from build123d import *

# Parameters (mm, degrees)
SKETCH2_W           = 127
SKETCH2_H           = 60
SKETCH2_W_2         = 105
SKETCH2_H_2         = 41
BOSS_EXTRUDE2_DEPTH = 8
SKETCH3_R           = 2.15
CUT_EXTRUDE1_DEPTH  = 5.159375
SKETCH4_W           = 11
SKETCH4_H           = 9.5
BOSS_EXTRUDE3_DEPTH = 25


with BuildPart() as part:
    # Sketch2 → Boss-Extrude2 (new body)
    with BuildSketch(Plane(origin=(0, 0, 0), x_dir=(1, 0, 0), z_dir=(0, 1, 0))):
        Rectangle(SKETCH2_W, SKETCH2_H)
        Rectangle(SKETCH2_W_2, SKETCH2_H_2, mode=Mode.SUBTRACT)
    extrude(amount=-BOSS_EXTRUDE2_DEPTH)

    # Sketch3 → Cut-Extrude1 (cut)
    with BuildSketch(Plane(origin=(0, 0, 0), x_dir=(1, 0, 0), z_dir=(0, 1, 0))):
        with Locations((5.055, -24.285)):
            Circle(SKETCH3_R)
        with Locations((-5.055, 24.285)):
            Circle(SKETCH3_R)
        with Locations((5.055, 24.285)):
            Circle(SKETCH3_R)
        with Locations((-5.055, -24.285)):
            Circle(SKETCH3_R)
    extrude(amount=-CUT_EXTRUDE1_DEPTH, mode=Mode.SUBTRACT)

    # Sketch4 → Boss-Extrude3 (add)
    with BuildSketch(Plane.XZ.offset(8)):
        with Locations((-58, 25.25)):
            Rectangle(SKETCH4_W, SKETCH4_H)
        with Locations((58, 25.25)):
            Rectangle(SKETCH4_W, SKETCH4_H)
        with Locations((58, -25.25)):
            Rectangle(SKETCH4_W, SKETCH4_H)
        with Locations((-58, -25.25)):
            Rectangle(SKETCH4_W, SKETCH4_H)
    extrude(amount=BOSS_EXTRUDE3_DEPTH)


solid = part.part
Design review of the part built by this model. Coordinates are the model's own, in mm. A direction names the side the tool comes from. Give positions to 0.01 mm unless a question says otherwise; leave off trailing zeros. Loops run counter-clockwise (first coordinate to the right, second up) from the corner with the lowest first, then second, coordinate; pieces in that order, holes last. Notation, with made-up numbers: (70.25, -8) -> (106.25, -8) arc R9 ccw to (106.25, -2) -> close; hole circle Ø5 at (46.5, 19). An arc over 180 degrees is marked (long way). One line per question, with ' | ' between items. Start each with the question number.
(1) We need section B-B (z = -17). State the section outline as (x, y) points, and give its area (3 significant figures).
(2) We need section D-D (y = -2.5). State the section outline as (x, z) points (3 decimals).
(3) We need section A-A (y = -10). State the section outline as (x, z) points.
(4) Draft analysis for pull direction Z (two halves, no side actions). For faces 4 (the face through (52.5, -4, 0)), 5 (the face through (63.5, -5, 0)), 6 (the face through (-1, -5, 30)), state which applies: +Z half, -Z half, draft (parallel to the pull), parting line (faces both ways), or undercut.
(5) For faces 1 (the face through (-58, -8, 0)), 2 (the face through (52.5, -20, -25)), 3 (the face through (5, -5.159, -24)), list the 3-axis set-ups (+Z, -Z, +X, -X, +Y, -Y) from which the entire face can be reached by the end or side of a thin tool; tool diameter is ignored.
(6) We need section C-C (x = -37.5). State the section outline as (y, z) points.
(7) For line 1 (X direction, y = -3, z = -7); line 2 (Z direction, x = -58, y = -26.5); line 3 (X direction, y = -4, z = -23), list the stretches that pass through material, from the lowest coordinate up.
(8) Insertion check: P1, Ø5.5, axis at x = -5.055, z = -24.285, coming from the -Y side; P2, Ø2.5, axis at x = -5.055, z = 24.285, coming from the +Y side. Each pin has a flat end and moves straight along its axis. Give the tip position at first contact, or say it passes through.
The answers:
1) outline: (-63.5, -8) -> (-52.5, -8) -> (-52.5, 0) -> (-63.5, 0) -> close; (52.5, -8) -> (63.5, -8) -> (63.5, 0) -> (52.5, 0) -> close | area: 176 mm^2
2) outline: (-63.5, -30) -> (63.5, -30) -> (63.5, 30) -> (-63.5, 30) -> close; hole (-52.5, -20.5) -> (52.5, -20.5) -> (52.5, 20.5) -> (-52.5, 20.5) -> close; hole circle Ø4.3 at (-5.055, -24.285); hole circle Ø4.3 at (-5.055, 24.285); hole circle Ø4.3 at (5.055, -24.285); hole circle Ø4.3 at (5.055, 24.285)
3) outline: (-63.5, -30) -> (-52.5, -30) -> (-52.5, -20.5) -> (-63.5, -20.5) -> close; (-63.5, 20.5) -> (-52.5, 20.5) -> (-52.5, 30) -> (-63.5, 30) -> close; (52.5, -30) -> (63.5, -30) -> (63.5, -20.5) -> (52.5, -20.5) -> close; (52.5, 20.5) -> (63.5, 20.5) -> (63.5, 30) -> (52.5, 30) -> close
4) face 4: undercut | face 5: draft | face 6: +Z half
5) face 1: +X, -X, -Y | face 2: +Z, -Z, -Y | face 3: +Y
6) outline: (-8, -30) -> (0, -30) -> (0, -20.5) -> (-8, -20.5) -> close; (-8, 20.5) -> (0, 20.5) -> (0, 30) -> (-8, 30) -> close
7) line 1: x = -63.5 to -52.5, 52.5 to 63.5 | line 2: z = -30 to -20.5, 20.5 to 30 | line 3: x = -63.5 to -6.78, -3.33 to 3.33, 6.78 to 63.5
8) P1: stops at y = -8 | P2: stops at y = -5.16
